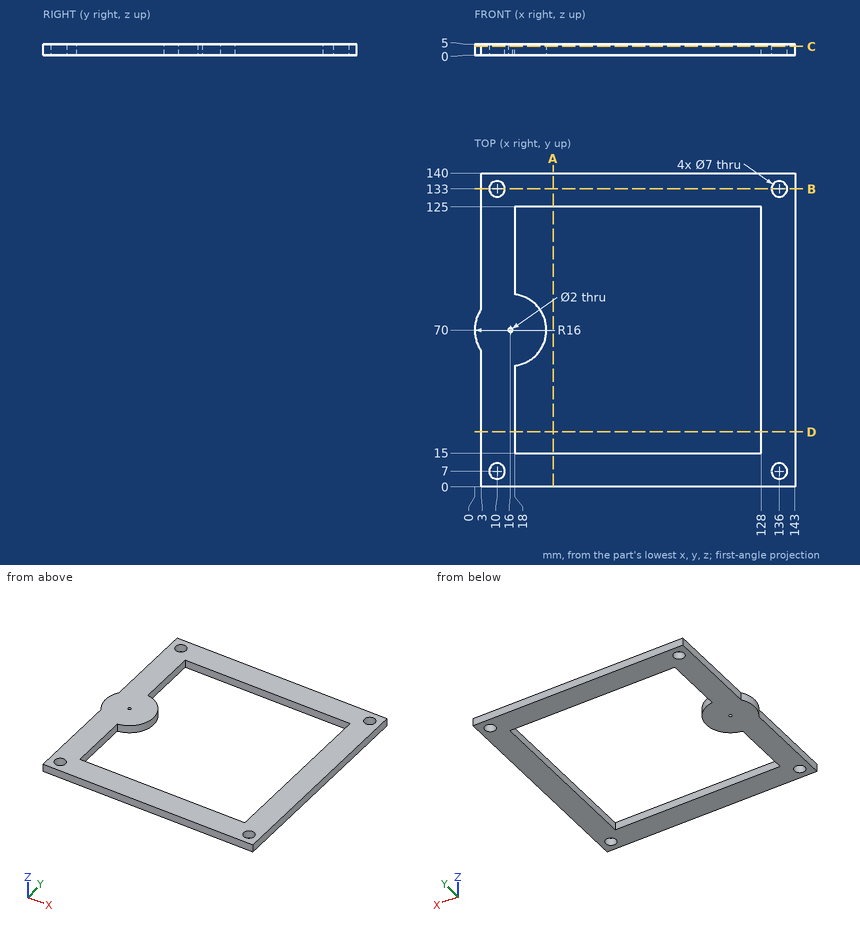
Can you work these out from the drawing? Everything is in mm from the part's minimum corner. Give positions to 0.01 mm unless a question says otherwise; leave off trailing zeros. Order: outer loops, then holes, each group sorted by start corner. A loop starts at its lowest first (then second) coordinate and runs counter-clockwise, first axis right, second up. Notation, with made-up numbers: M 7,-8.75 L 41,-8.75 A11 ccw 41,11.25 Z; hole C -16,56 d4. An arc over 180 degrees is marked long. One line per question, with ' | ' between items.
1. I want a section at B-B (y = 133). List the corners of the cut face in (x, z) for me, and give its area (3 significant figures).
Results:
outline: M 3,0 L 6.5,0 L 6.5,5 L 3,5 Z; M 13.5,0 L 132.5,0 L 132.5,5 L 13.5,5 Z; M 139.5,0 L 143,0 L 143,5 L 139.5,5 Z | area: 630 mm²
2. I want a section at A-A (x = 35). List the corners of the cut face in (y, z) for me, and give its area (3 significant figures).
Results:
outline: M 0,0 L 15,0 L 15,5 L 0,5 Z; M 125,0 L 140,0 L 140,5 L 125,5 Z | area: 150 mm²
3. If I drill on line 1 (X direction, y = 70, z = 3.4); line 2 (X direction, y = 133, z = 4); line 3 (X direction, y = 117, z = 0.75), over which ranges is the centre line in solid material (lowest first)?
Results:
line 1: 0 to 15, 17 to 32, 128 to 143 | line 2: 3 to 6.5, 13.5 to 132.5, 139.5 to 143 | line 3: 3 to 18, 128 to 143
4. I want a section at C-C (z = 3.95). List the corners of the cut face in (x, y) for me, and give its area (3 significant figures).
Results:
outline: M 3,0 L 143,0 L 143,140 L 3,140 L 3,79.33 A16 ccw 3,60.67 Z; hole C 10,7 d7; hole C 10,133 d7; hole C 16,70 d2; hole M 18,15 L 128,15 L 128,125 L 18,125 L 18,85.87 A16 cw 18,54.13 Z; hole C 136,7 d7; hole C 136,133 d7 | area: 7,720 mm²
5. I want a section at D-D (y = 24.5). List the corners of the cut face in (x, z) for me.
Results:
outline: M 3,0 L 18,0 L 18,5 L 3,5 Z; M 128,0 L 143,0 L 143,5 L 128,5 Z
6. I'm going to push flat-ended pins straight in: pin 1 (1.5 mm diameter, centred on y = 121.5, z = 2.5, fed in from -X); pin 2 (1.5 mm diameter, centred on y = 64.5, z = 3, fed in from -X). Where does each tip first touch, or does it pass through?
Results:
pin 1: x = 3 | pin 2: x = 0.72
